The model under review builds one solid part; all positions refer to its coordinate system, in mm. Face numbers are marked on the shaded views. A direction names the side the tool comes from. Give positions to 0.01 mm unless a question says otherwise; leave off trailing zeros. Loops run counter-clockwise (first coordinate to the right, second up) from the corner with the lowest first, then second, coordinate; pieces in that order, holes last. Notation, with made-up numbers: M 88.5,78.25 L 106.5,78.25 A29 ccw 106.5,104.25 Z; hole C 59,9.5 d3. An arc over 180 degrees is marked long. One line per item, written item: value. Start each with the question number.
Q1. To check wall thickness, follow line 1 along Y through (x, z) = (0, 0.95); line 2 along Z through (x, y) = (0.5, -9.5). State the ranges of each line that lie inside material, in increasing order. Write a range as from..to.
Q2. For pin 1 (0.6 mm diameter, centred on x = -10.5, y = -0.5, fed in from +Z); pin 2 (1.4 mm diameter, centred on x = 11.5, z = 2, fed in from -Y); pin 3 (0.6 mm diameter, centred on y = 10.5, z = 2, fed in from +X), all flat-tipped, find the tip position at first contact; note any pin that passes through.
Q3. For the marked faces 1 and 2, list the 3-axis set-ups (+Z, -Z, +X, -X, +Y, -Y) from which the entire face can be reached by the end or side of a thin tool; tool diameter is ignored.
Q4. We need section D-D on z = 0.8. Write out the cut boundary in (x, y), plus the area to 3 significant figures.
Q5. We need section A-A on x = 0. Write out the cut boundary in (y, z), plus the area to 3 significant figures.
Q6. We need section C-C on x = 5.5. Write out the cut boundary in (y, z), plus the area to 3 significant figures.
Q7. Mouldability with a two-part tool opening along Y and no side actions: class the marked faces 3, 4, 5 and 6 as released by +Y, released by -Y, zero draft, split by the parting line, or undercut.
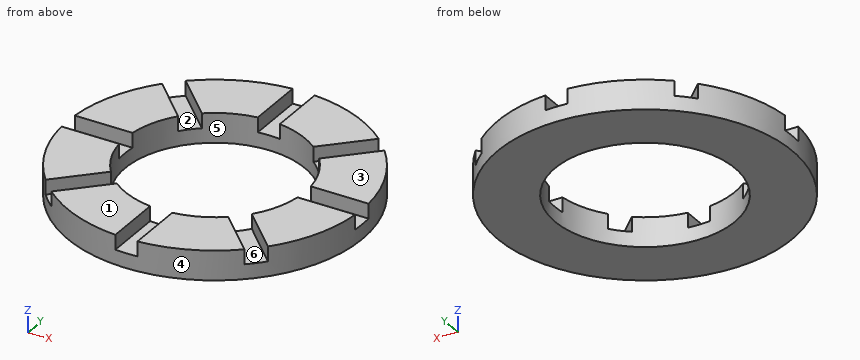
```python
from build123d import *

# Parameters (mm, degrees)
F0_R     = 12.7
F0_R_2   = 7.747
F1_DEPTH = 2.54
F3_DEPTH = 1.27
F4_W     = 1.905
F4_H     = 11.7475
F4_W_2   = 11.7475
F4_H_2   = 1.905
F5_DEPTH = 1.27


with BuildPart() as f1:
    # F0 (on Top) → F1 (new body)
    with BuildSketch(Plane.XY):
        Circle(F0_R)
        Circle(F0_R_2, mode=Mode.SUBTRACT)
    extrude(amount=F1_DEPTH)

    # F2 (on face) → F3 (cut)
    with BuildSketch(Plane.XY.offset(2.54)):
        Polygon((0, 1.27), (0, 0), (6.35, 6.35), (9.698677, 9.698677), (8.428677, 9.698677), align=None)
        Polygon((-1.27, 0), (0, 0), (-6.35, 6.35), (-9.698677, 9.698677), (-9.698677, 8.428677), align=None)
        Polygon((1.27, 0), (0, 0), (6.35, -6.35), (9.698677, -9.698677), (9.698677, -8.428677), align=None)
        Polygon((0, -1.27), (0, 0), (-6.35, -6.35), (-9.698677, -9.698677), (-8.428677, -9.698677), align=None)
        Polygon((6.35, 6.35), (0, 0), (1.27, 0), (9.698677, 8.428677), (9.698677, 9.698677), align=None)
        Polygon((-6.35, 6.35), (0, 0), (0, 1.27), (-8.428677, 9.698677), (-9.698677, 9.698677), align=None)
        Polygon((6.35, -6.35), (0, 0), (0, -1.27), (8.428677, -9.698677), (9.698677, -9.698677), align=None)
        Polygon((-6.35, -6.35), (0, 0), (-1.27, 0), (-9.698677, -8.428677), (-9.698677, -9.698677), align=None)
    extrude(amount=-F3_DEPTH, mode=Mode.SUBTRACT)

    # F4 (on face) → F5 (cut)
    with BuildSketch(Plane.XY.offset(2.54)):
        with Locations((0, -6.82625)):
            Rectangle(F4_W, F4_H)
        with Locations((6.82625, 0)):
            Rectangle(F4_W_2, F4_H_2)
        with Locations((-6.82625, 0)):
            Rectangle(F4_W_2, F4_H_2)
        with Locations((0, 6.82625)):
            Rectangle(F4_W, F4_H)
    extrude(amount=-F5_DEPTH, mode=Mode.SUBTRACT)


solid = f1.part
```
Solved:
1. line 1: -12.7..-7.75, 7.75..12.7
1. line 2: 0..1.27
2. pin 1: z = 1.27
2. pin 2: y = -6.68
2. pin 3: x = 7.57
3. face 1: +Z, +X, -X, +Y, -Y
3. face 2: +Z
4. outline: C 0,0 d25.4; hole C 0,0 d15.49
4. area: 318 mm2
5. outline: M -12.7,0 L -7.75,0 L -7.75,1.27 L -12.7,1.27 Z; M 7.75,0 L 12.7,0 L 12.7,1.27 L 7.75,1.27 Z
5. area: 12.6 mm2
6. outline: M -11.45,0 L -5.46,0 L -5.46,1.27 L -6.77,1.27 L -6.77,2.54 L -11.45,2.54 Z; M 5.46,0 L 11.45,0 L 11.45,2.54 L 6.77,2.54 L 6.77,1.27 L 5.46,1.27 Z
6. area: 27.1 mm2
7. face 3: zero draft
7. face 4: split by the parting line
7. face 5: undercut
7. face 6: undercut
